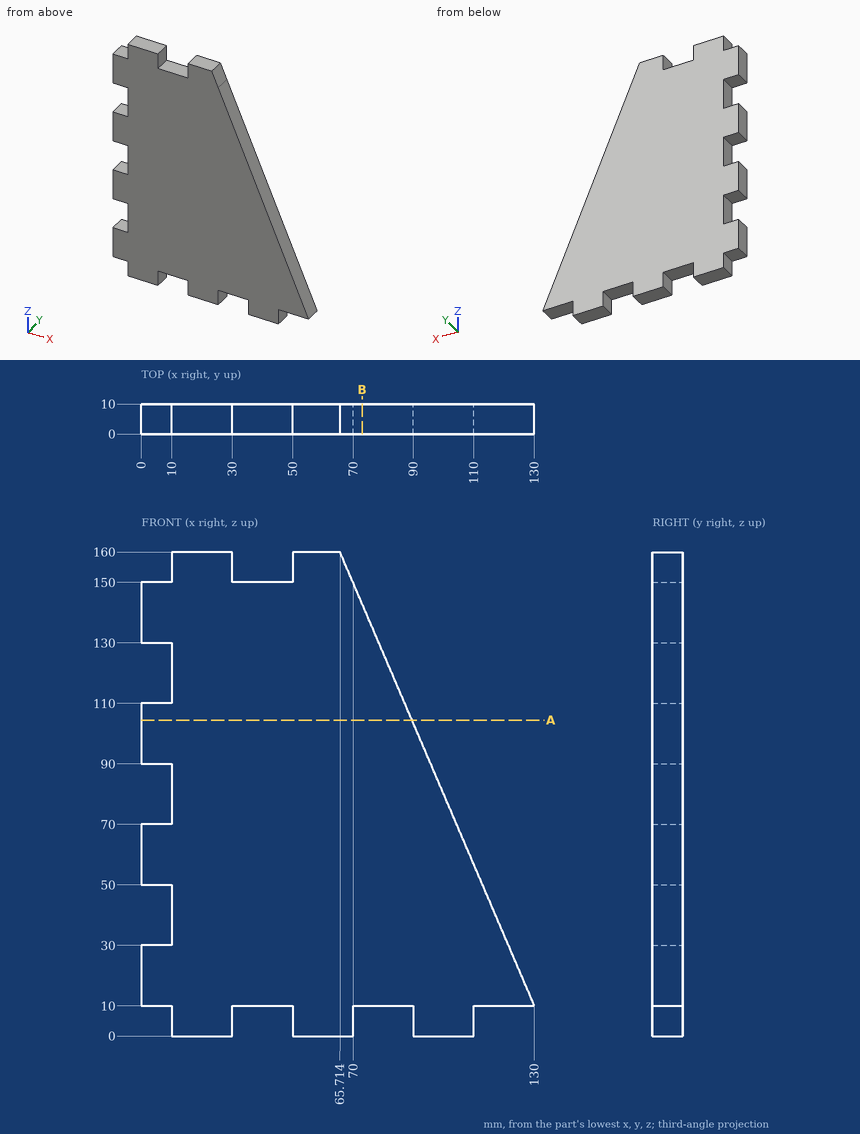
Verification items for this drawing (mm, ordinates from the low corner). Give positions to 0.01 mm unless a question says otherwise; leave off trailing zeros. Loops run counter-clockwise (first coordinate to the right, second up) from the corner with the lowest first, then second, coordinate; pieces in that order, holes last. Notation, with made-up numbers: M 19.5,-26.75 L 40.5,-26.75 A27 ccw 40.5,3.25 Z; hole C 8.5,-15.5 d7. An arc over 180 degrees is marked long. Answer in a Markdown table with one row per item.
1) Cross-section at A-A (z = 104.5). Enter the section's corners in (x, y), plus the area to 3 significant figures.
Solutions:
| item | result |
|---|---|
| outline | M 0,0 L 89.5,0 L 89.5,10 L 0,10 Z |
| area | 895 mm^2 |
2) Thickness scan on line 1 (Z direction, x = 9, y = 3.25); line 2 (Z direction, x = 34, y = 5.5); line 3 (X direction, y = 2.25, z = 153) (1 decimal). Record the ranges inside material, lowest first.
Solutions:
| item | result |
|---|---|
| line 1 | z = 10 to 30, 50 to 70, 90 to 110, 130 to 150 |
| line 2 | z = 10 to 150 |
| line 3 | x = 10 to 30, 50 to 68.7 |
3) Cross-section at B-B (x = 73). Enter the section's corners in (y, z), plus the area to 3 significant figures.
Solutions:
| item | result |
|---|---|
| outline | M 0,10 L 10,10 L 10,143 L 0,143 Z |
| area | 1,330 mm^2 |
4) Depth check by flat-ended pin: pin 1 (5 mm diameter, centred on y = 7, z = 2.5, fed in from -X); pin 2 (6 mm diameter, centred on x = 86.5, y = 8, fed in from -Z); pin 3 (5 mm diameter, centred on y = 6, z = 3, fed in from +X). Enter the tip coordinate at first touch or a pass-through.
Solutions:
| item | result |
|---|---|
| pin 1 | stops at x = 10 |
| pin 2 | stops at z = 10 |
| pin 3 | stops at x = 110 |
